```python
from build123d import *

# Parameters (mm, degrees)
F0_R     = 2.9651856051
F1_DEPTH = 10
F2_DEPTH = 35
F3_D     = 6


with BuildPart() as f1:
    # F0 (on Front) → F1 (new body)
    with BuildSketch(Plane.XZ):
        with BuildLine():
            Line((1, 50), (-1, 50))
            ThreePointArc((-1, 50), (-4.5355339059, 48.5355339059), (-6, 45))
            Line((-6, 45), (-6, -45))
            ThreePointArc((-6, -45), (-4.5355339059, -48.5355339059), (-1, -50))
            Line((-1, -50), (1, -50))
            ThreePointArc((1, -50), (4.5355339059, -48.5355339059), (6, -45))
            Line((6, -45), (6, 45))
            ThreePointArc((6, 45), (4.5355339059, 48.5355339059), (1, 50))
        make_face()
        with Locations((0, -45)):
            Circle(F0_R, mode=Mode.SUBTRACT)
        with Locations((0, -45)):
            Circle(F0_R)
    extrude(amount=F1_DEPTH)

    # F0 (on Front) → F2 (join)
    with BuildSketch(Plane.XZ):
        with Locations((0, -45)):
            Circle(F0_R)
    extrude(amount=F2_DEPTH)

    # F3 (through all)
    with Locations(Plane(origin=(0, 0, 0), x_dir=(1, 0, 0), z_dir=(0, 1, 0))):
        with Locations((0, -45)):
            Hole(F3_D / 2)


solid = f1.part
```
The model under review builds one solid part; all positions refer to its coordinate system, in mm. A direction names the side the tool comes from. Give positions to 0.01 mm unless a question says otherwise; leave off trailing zeros. Write each loop counter-clockwise with the first axis right and the second up, starting at its lowest first coordinate (ties: lowest second). Pieces come first, ordered by that corner, then holes. Notation, with made-up numbers: (-3, 4) - (36, 4) arc R23 cw to (36, 27) - close; hole circle Ø10 at (85, -5.75). An arc over 180 degrees is marked (long way). Answer in a Markdown table with one row per item. Add a question column.
1. Wall thickness on line 1 along Z through (x, y) = (0, -7.25); line 2 along X through (y, z) = (-2.75, 45); line 3 along Y through (x, z) = (-4.5, -19): over which ranges is each line inside the solid? List them lowest first. Write a range as [from, to].
2. Tool access review of faces 5 (the flat face through (0, -5, 50)), 6 (the cylindrical face through (-0.643, -22.325, -47.895)): name each direction out of +Z, -Z, +X, -X, +Y, -Y from which nothing blocks a thin tool from reaching the whole face with its end or side.
3. Draft analysis for pull direction Z (two halves, no side actions). For faces 1 (the cylindrical face through (-4, -5, 49)), 2 (the cylindrical face through (4, -5, -49)), 3 (the cylindrical face through (0, -5, 42)), 4 (the flat face through (0, 0, 1)), state which applies: +Z half, -Z half, draft (parallel to the pull), parting line (faces both ways), or undercut.
4. Insertion check: P1, Ø3.5, axis at x = 0, z = 45, coming from the -Y side; P2, Ø6, axis at x = -0.5, z = -17.5, coming from the -Y side. Each pin has a flat end and moves straight along its axis. Give the tip position at first contact, or say it passes through.
5. We need section B-B on y = -7. Write out the cut boundary in (x, z).
6. We need section C-C on z = 43. Write out the cut boundary in (x, y), then the cut area to 3 significant figures.
7. We need section D-D on z = 31.5. Write out the cut boundary in (x, y), then the cut area to 3 significant figures.
8. We need section A-A on x = 0. Write out the cut boundary in (y, z), then the cut area to 3 significant figures.
Ans:
| question | item | result |
|---|---|---|
| 1 | line 1 | z = [-50, 42], [48, 50] |
| 1 | line 2 | x = [-6, -3], [3, 6] |
| 1 | line 3 | y = [-10, 0] |
| 2 | face 5 | +Z, +X, -X, +Y, -Y |
| 2 | face 6 | -Y |
| 3 | face 1 | +Z half |
| 3 | face 2 | -Z half |
| 3 | face 3 | undercut |
| 3 | face 4 | draft |
| 4 | P1 | passes through |
| 4 | P2 | stops at y = -10 |
| 5 | outline | (-6, -45) arc R5 ccw to (-1, -50) - (1, -50) arc R5 ccw to (6, -45) - (6, 45) arc R5 ccw to (1, 50) - (-1, 50) arc R5 ccw to (-6, 45) - close; hole circle Ø6 at (0, 45) |
| 6 | outline | (-6, -10) - (-2.24, -10) - (-2.24, 0) - (-6, 0) - close; (2.24, -10) - (6, -10) - (6, 0) - (2.24, 0) - close |
| 6 | area | 75.3 mm^2 |
| 7 | outline | (-6, -10) - (6, -10) - (6, 0) - (-6, 0) - close |
| 7 | area | 120 mm^2 |
| 8 | outline | (-35, -47.97) - (-10, -47.97) - (-10, -50) - (0, -50) - (0, 42) - (-10, 42) - (-10, -42.03) - (-35, -42.03) - close; (-10, 48) - (0, 48) - (0, 50) - (-10, 50) - close |
| 8 | area | 1,090 mm^2 |
